from build123d import *

# Parameters (mm, degrees)
BOSS_EXTRUDE1_DEPTH  = 15
SKETCH3_W            = 340.59039901
SKETCH3_H            = 15
BOSS_EXTRUDE2_DEPTH  = 8
M6_CLEARANCE_HOLE1_D = 6.6


with BuildPart() as part:
    # Sketch1 → Boss-Extrude1 (new, symmetric)
    with BuildSketch(Plane.XY):
        with BuildLine():
            Line((-132.3, 16), (132.3, 16))
            ThreePointArc((132.3, 16), (142.040182864, 12.693653445), (147.754813221, 4.141104722))
            Line((147.754813221, 4.141104722), (155.295199505, -24))
            Line((155.295199505, -24), (170.295199505, -24))
            Line((170.295199505, -24), (170.295199505, -32))
            Line((170.295199505, -32), (-170.295199505, -32))
            Line((-170.295199505, -32), (-170.295199505, -24))
            Line((-170.295199505, -24), (-155.295199505, -24))
            Line((-155.295199505, -24), (-147.754813221, 4.141104722))
            ThreePointArc((-147.754813221, 4.141104722), (-142.040182864, 12.693653445), (-132.3, 16))
        make_face()
        with BuildLine():
            Line((-132.3, 10), (132.3, 10))
            ThreePointArc((132.3, 10), (142.3, 0), (132.3, -10))
            Line((132.3, -10), (-132.3, -10))
            ThreePointArc((-132.3, -10), (-142.3, 0), (-132.3, 10))
        make_face(mode=Mode.SUBTRACT)
    extrude(amount=BOSS_EXTRUDE1_DEPTH, both=True)

    # Sketch3 → Boss-Extrude2 (add)
    with BuildSketch(Plane.XZ.offset(32)):
        with Locations((0, 22.5)):
            Rectangle(SKETCH3_W, SKETCH3_H)
    boss_extrude2 = extrude(amount=-BOSS_EXTRUDE2_DEPTH)

    # Mirror1: Boss-Extrude2 across plane
    add(boss_extrude2.mirror(Plane.XY))

    # M6 Clearance Hole1 (through all)
    with Locations(Plane(origin=(-162.795199505, -24, -22.5), x_dir=(1, 0, 0), z_dir=(0, 1, 0))):
        with Locations((0, 0), (0, -45), (81.397599753, -45), (81.397599753, 0), (162.795199505, -45), (162.795199505, 0), (244.192799257, -45), (244.192799257, 0), (325.59039901, 0), (325.59039901, -45)):
            Hole(M6_CLEARANCE_HOLE1_D / 2)


solid = part.part
Can you work these out from the model? Positions are in its coordinate system, mm. A direction names the side the tool comes from. Coordinates: 2 decimals unless noted, no trailing zeros. Loops run counter-clockwise (first coordinate to the right, second up) from the corner with the lowest first, then second, coordinate; pieces in that order, holes last. Notation, with made-up numbers: (69, 74.5) - (104, 74.5) arc R20 ccw to (104, 107.5) - close; hole circle Ø1 at (49, 86). An arc over 180 degrees is marked (long way). Answer as a JSON object with one key per item and string values. Group by question number.
Item 1: If we section it at D-D (y = -6.5): List the corners of the cut face in (x, z) for me, plus the area to 3 significant figures.
Item 2: For pin 1 (7.5 mm diameter, centred on x = -162.8, z = 22.5, fed in from +Y); pin 2 (6 mm diameter, centred on x = 39.5, y = -23.5, fed in from -Z); pin 3 (4 mm diameter, centred on x = 162.8, z = -22.5, fed in from +Y); pin 4 (2 mm diameter, centred on y = -3, z = 15.5, fed in from -X), each with a flat end and sliding along its axis, tell me the tip position at first contact or that it passes through.
Item 3: If we section it at A-A (x = -101): List the corners of the cut face in (y, z) for me, plus the area to 3 significant figures.
Item 4: If I drill on L1, parallel to X at y = -29.75, z = 22.5; L2, parallel to Z at x = 0, y = -28.5; L3, parallel to Y at x = -28, z = 11, over which ranges is the centre line in solid material (lowest first)? Write a range as from..to.
Item 5: If we mould it in two halves opening along Z, with no side actions, what happens to faces 1 (the face through (0.72, -28.06, 25.72)), 2 (the face through (-2, -28, 30)), 3 (the face through (-2.4, -24, 19.6))? For each: released by +Z, released by -Z, zero draft, split by the parting line, or undercut.
Item 6: If we section it at B-B (x = 0): List the corners of the cut face in (y, z) for me.
Item 7: If we section it at C-C (z = -22.5): List the corners of the cut face in (x, y) for me, plus the area to 3 significant figures.
Item 8: On a 3-axis mill with a long thin cutter (end or side, diameter ignored), from which of +Z, -Z, +X, -X, +Y, -Y can I reach the whole of each face in a straight line? I mean faces 4 (the face through (142.3, 0.2, 0.2)), 5 (the face through (2, -13, 15)), 6 (the face through (2, -13, -15)). Say none if no direction works.
Returned:
{
 "1": {"outline": "(-150.61, -15) - (-139.9, -15) - (-139.9, 15) - (-150.61, 15) - close; (139.9, -15) - (150.61, -15) - (150.61, 15) - (139.9, 15) - close", "area": "642 mm²"},
 "2": {"pin 1": "stops at y = -24", "pin 2": "stops at z = -30", "pin 3": "passes through", "pin 4": "stops at x = -149.9"},
 "3": {"outline": "(-32, -30) - (-24, -30) - (-24, -15) - (-10, -15) - (-10, 15) - (-24, 15) - (-24, 30) - (-32, 30) - close; (10, -15) - (16, -15) - (16, 15) - (10, 15) - close", "area": "1,080 mm²"},
 "4": {"L1": "x = -170.3..-166.1, -159.5..-84.7, -78.1..-3.3, 3.3..78.1, 84.7..159.5, 166.1..170.3", "L2": "z = -30..-25.8, -19.2..19.2, 25.8..30", "L3": "y = -32..-10, 10..16"},
 "5": {"face 1": "undercut", "face 2": "released by +Z", "face 3": "zero draft"},
 "6": {"outline": "(-32, -30) - (-24, -30) - (-24, -25.8) - (-32, -25.8) - close; (-32, -19.2) - (-24, -19.2) - (-24, -15) - (-10, -15) - (-10, 15) - (-24, 15) - (-24, 19.2) - (-32, 19.2) - close; (-32, 25.8) - (-24, 25.8) - (-24, 30) - (-32, 30) - close; (10, -15) - (16, -15) - (16, 15) - (10, 15) - close"},
 "7": {"outline": "(-170.3, -32) - (-166.1, -32) - (-166.1, -24) - (-170.3, -24) - close; (-159.5, -32) - (-84.7, -32) - (-84.7, -24) - (-159.5, -24) - close; (-78.1, -32) - (-3.3, -32) - (-3.3, -24) - (-78.1, -24) - close; (3.3, -32) - (78.1, -32) - (78.1, -24) - (3.3, -24) - close; (84.7, -32) - (159.5, -32) - (159.5, -24) - (84.7, -24) - close; (166.1, -32) - (170.3, -32) - (170.3, -24) - (166.1, -24) - close", "area": "2,460 mm²"},
 "8": {"face 4": "+Z, -Z", "face 5": "+Z, +X, -X, +Y", "face 6": "-Z, +X, -X, +Y"}
}
